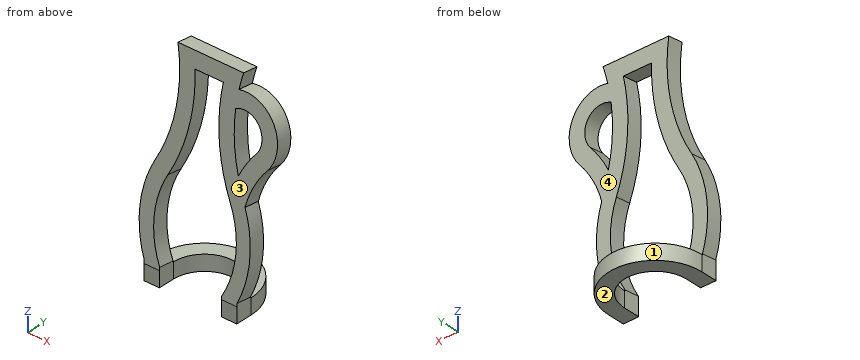
```python
from build123d import *

# Parameters (mm, degrees)
F4_DEPTH = 25.4
F6_DEPTH = 25.4


with BuildPart() as f4:
    # F3 (on offset) → F4 (new body)
    with BuildSketch(Plane.XY):
        with BuildLine():
            Line((-76.2, 26.9875), (-76.2, 0))
            Line((-76.2, 0), (-50.8, 0))
            Line((-50.8, 0), (-50.8, 26.9875))
            ThreePointArc((-50.8, 26.9875), (0, 77.7875), (50.8, 26.9875))
            Line((50.8, 26.9875), (50.8, 0))
            Line((50.8, 0), (76.2, 0))
            Line((76.2, 0), (76.2, 26.9875))
            ThreePointArc((76.2, 26.9875), (0, 103.1875), (-76.2, 26.9875))
        make_face()
    extrude(amount=-F4_DEPTH)

    # F5 (on line) → F6 (join)
    with BuildSketch(Plane(origin=(0, 0, 0), x_dir=(-1, 0, 0), z_dir=(0, 0.9925461516, -0.1218693434))):
        with BuildLine():
            ThreePointArc((-75.0903723478, 138.827645489), (-90.0403532632, 71.9142183688), (-76.2, 4.7625))
            Line((-76.2, 4.7625), (-76.2, 0))
            Line((-76.2, 0), (-50.8, 0))
            Line((-50.8, 0), (-50.8, 4.7625))
            ThreePointArc((-50.8, 4.7625), (-67.3023617732, 70.0071639204), (-51.3841879778, 135.3968103272))
            ThreePointArc((-51.3841879778, 135.3968103272), (-25.0859353678, 212.368668197), (-23.2117561056, 293.6875002493))
            Line((-23.2117561056, 293.6875002493), (0, 293.6875002493))
            Line((0, 293.6875002493), (23.1415493167, 293.6875002493))
            ThreePointArc((23.1415493167, 293.6875002493), (24.7523028396, 211.7684987185), (51.1552849917, 134.2043325579))
            ThreePointArc((51.1552849917, 134.2043325579), (66.8742650231, 69.439784083), (50.8, 4.7625))
            Line((50.8, 4.7625), (50.8, 0))
            Line((50.8, 0), (76.2, 0))
            Line((76.2, 0), (76.2, 4.7625))
            ThreePointArc((76.2, 4.7625), (90.7935935425, 75.6597014149), (73.6577047551, 145.9857098073))
            ThreePointArc((73.6577047551, 145.9857098073), (47.6694306232, 230.702066542), (54.0150973414, 319.0874952316))
            Line((54.0150973414, 319.0874952316), (0, 319.0874952316))
            Line((0, 319.0874952316), (-54.0150973414, 319.0874952316))
            ThreePointArc((-54.0150973414, 319.0874952316), (-51.0804025225, 306.5319685143), (-48.8205663921, 293.8376065574))
            ThreePointArc((-48.8205663921, 293.8376065574), (-108.938602772, 268.4421399471), (-106.0506710111, 203.2442268465))
            ThreePointArc((-106.0506710111, 203.2442268465), (-86.3813942483, 173.049340693), (-75.0903723478, 138.827645489))
        make_face()
        with BuildLine():
            ThreePointArc((-46.2746955842, 266.2427872527), (-48.9959426673, 220.834025793), (-60.1912430767, 176.7429149913))
            ThreePointArc((-60.1912430767, 176.7429149913), (-71.5917023099, 198.9100774911), (-86.1994937771, 219.1082455385))
            ThreePointArc((-86.1994937771, 219.1082455385), (-84.8490348444, 258.4405568096), (-46.2746955842, 266.2427872527))
        make_face(mode=Mode.SUBTRACT)
    extrude(amount=F6_DEPTH)


solid = f4.part
```
Can you work these out from the model? Positions are in its coordinate system, mm. Face numbers are marked on the shaded views. Coordinates: 2 decimals unless noted, no trailing zeros. Loops run counter-clockwise (first coordinate to the right, second up) from the corner with the lowest first, then second, coordinate; pieces in that order, holes last. Notation, with made-up numbers: (-33.75, 88.25) - (-3.75, 88.25) arc R26 ccw to (-3.75, 106.25) - close; hole circle Ø9 at (-10, 18.25). An arc over 180 degrees is marked (long way). Use a Markdown table: item, result.
Item 1: I want a section at B-B on z = 192.5. Give the number of separate pieces and of enclosed holes in the cut face, and give its area (3 significant figures).
Numbers:
| item | result |
|---|---|
| separate pieces | 3 |
| enclosed holes | 0 |
| area | 2,100 mm2 |
Item 2: I want a section at C-C on x = -27. Please give me the cut outline in (y, z).
Numbers:
| item | result |
|---|---|
| outline | (24.43, 198.93) - (49.64, 195.83) - (64.1, 313.61) - (38.89, 316.71) - close; (70.02, -25.4) - (98.24, -25.4) - (98.24, 0) - (70.02, 0) - close |
Item 3: If I drill on probe 1 along X at (y, z) = (49.5, 246.5); probe 2 along Z at (x, y) = (62.5, 68.5); probe 3 along X at (y, z) = (19.5, 105.5), over which ranges is the centre line in solid material (lowest first)? Write a range as from..to.
Numbers:
| item | result |
|---|---|
| probe 1 | x = -46.24..-20.83, 21.09..46.24, 89.69..116.33 |
| probe 2 | z = -25.4..0 |
| probe 3 | x = -87.2..-61.81, 62.46..85.91 |
Item 4: We'd pull the mould along Z, two halves only. Please class the marked faces 1, 2, 3 and 4: released by +Z, released by -Z, zero draft, split by the parting line, or undercut.
Numbers:
| item | result |
|---|---|
| face 1 | zero draft |
| face 2 | released by -Z |
| face 3 | released by +Z |
| face 4 | undercut |
Item 5: Will these pins go through, and if not, where does the flat tip stop? pin 1 (8 mm diameter, centred on y = 11, z = -14, fed in from -X); pin 2 (13.5 mm diameter, centred on y = 18, z = -4.5, fed in from +X); pin 3 (23.5 mm diameter, centred on x = 15.5, y = 56, fed in from +Z).
Numbers:
| item | result |
|---|---|
| pin 1 | stops at x = -76.2 |
| pin 2 | stops at x = 76.2 |
| pin 3 | stops at z = 316.05 |
Item 6: I want a section at A-A on x = 0. Please give me the cut outline in (y, z).
Numbers:
| item | result |
|---|---|
| outline | (35.79, 291.5) - (61, 288.4) - (64.1, 313.61) - (38.89, 316.71) - close; (77.79, -25.4) - (103.19, -25.4) - (103.19, 0) - (77.79, 0) - close |
